Verification items for the finished model (mm, model axes). A direction names the side the tool comes from. Coordinates: 2 decimals unless noted, no trailing zeros. Order: outer loops, then holes, each group sorted by start corner. A loop starts at its lowest first (then second) coordinate and runs counter-clockwise, first axis right, second up.
Q1. Set-up check for faces 4 (the flat face through (0, 0, 0)), 5 (the cylindrical face through (0.45, 5.91, 1.43)): record each of +Z, -Z, +X, -X, +Y, -Y from which the full face is reachable in a straight line by a thin tool's end or side.
Q2. Cross-section at A-A, the plane x = 0. Record the boundary of the cut face in (y, z), and give its area (3 significant figures).
Q3. Depth check by flat-ended pin: P1, Ø2.5, axis at x = -0.5, z = -0.5, coming from the +Y side; P2, Ø1.5, axis at x = -1.5, y = 10.5, coming from the -Z side; P3, Ø1, axis at x = 1.5, y = 6, coming from the -Z side. Enter the tip coordinate at first touch or a pass-through.
Q4. Thickness scan on line 1 (X direction, y = 11.2, z = 0); line 2 (X direction, y = 6, z = 0); line 3 (Z direction, x = -0.5, y = 9.5). Record the ranges inside material, lowest first.
Q5. Cross-section at B-B, the plane z = 0. Record the boundary of the cut face in (x, y), and give its area (3 significant figures).
Q6. Draft check along X on faces 1 (the flat face through (0, 3.5, 0)), 2 (the cylindrical face through (1.802, 6.17, 5.723)), 3 (the flat face through (4, 12, -4)). Enter one of: pulls with the +X half, pulls with the -X half, needs draft (parallel to the pull), parting line crosses it, or undercut.
Q7. Cross-section at C-C, the plane y = 9.75. Record the boundary of the cut face in (x, z), and give its area (3 significant figures).
from build123d import *

# Parameters (mm, degrees)
SKETCH1_R           = 6
BOSS_EXTRUDE1_DEPTH = 12
SKETCH2_R           = 5
CUT_EXTRUDE1_DEPTH  = 3
CHAMFER1_SIZE       = 0.5


with BuildPart() as part:
    # Sketch1 → Boss-Extrude1 (new body)
    with BuildSketch(Plane(origin=(0, 0, 0), x_dir=(1, 0, 0), z_dir=(0, 1, 0))):
        with Locations(Location((0, 0, 0), (0, 0, 270))):
            Circle(SKETCH1_R)
    extrude(amount=BOSS_EXTRUDE1_DEPTH)

    # Sketch2 → Cut-Extrude1 (cut)
    with BuildSketch(Plane(origin=(0, 12, 0), x_dir=(1, 0, 0), z_dir=(0, 1, 0))):
        with Locations(Location((0, 0, 0), (0, 0, 270))):
            Circle(SKETCH2_R)
    extrude(amount=-CUT_EXTRUDE1_DEPTH, mode=Mode.SUBTRACT)

    # Sketch3 → Cut-Revolve1 (revolve, cut)
    with BuildSketch(Plane.XY, mode=Mode.PRIVATE) as cut_revolve1_sk:
        Polygon((-5, 9), (-1.5, 8.382855568), (-1.5, 3.5), (0, 3.5), (0, 9), align=None)
    revolve(cut_revolve1_sk.sketch.rotate(Axis((0, 3.5, 0), (0, 1, 0)), 90), axis=Axis((0, 3.5, 0), (0, 1, 0)), mode=Mode.SUBTRACT)

    # Chamfer1
    chamfer1_edges = [part.edges().sort_by_distance(p)[0] for p in [
        (0, 0, -6),
    ]]
    chamfer(chamfer1_edges, length=CHAMFER1_SIZE)


solid = part.part
Check values:
1. face 4: +Z, -Z, +X, -X, -Y
1. face 5: +Y
2. outline: (0, -5.5) - (0.5, -6) - (12, -6) - (12, -5) - (9, -5) - (8.38, -1.5) - (3.5, -1.5) - (3.5, 1.5) - (8.38, 1.5) - (9, 5) - (12, 5) - (12, 6) - (0.5, 6) - (0, 5.5) - close
2. area: 95.1 mm2
3. P1: stops at y = 8.46
3. P2: stops at z = -5.95
3. P3: stops at z = -5.92
4. line 1: x = -6 to -5, 5 to 6
4. line 2: x = -6 to -1.5, 1.5 to 6
4. line 3: z = -5.98 to -4.97, 4.97 to 5.98
5. outline: (-6, 0.5) - (-5.5, 0) - (5.5, 0) - (6, 0.5) - (6, 12) - (5, 12) - (5, 9) - (1.5, 8.38) - (1.5, 3.5) - (-1.5, 3.5) - (-1.5, 8.38) - (-5, 9) - (-5, 12) - (-6, 12) - close
5. area: 95.1 mm2
6. face 1: undercut
6. face 2: parting line crosses it
6. face 3: needs draft
7. outline: circle Ø12 at (0, 0); hole circle Ø10 at (0, 0)
7. area: 34.6 mm2
